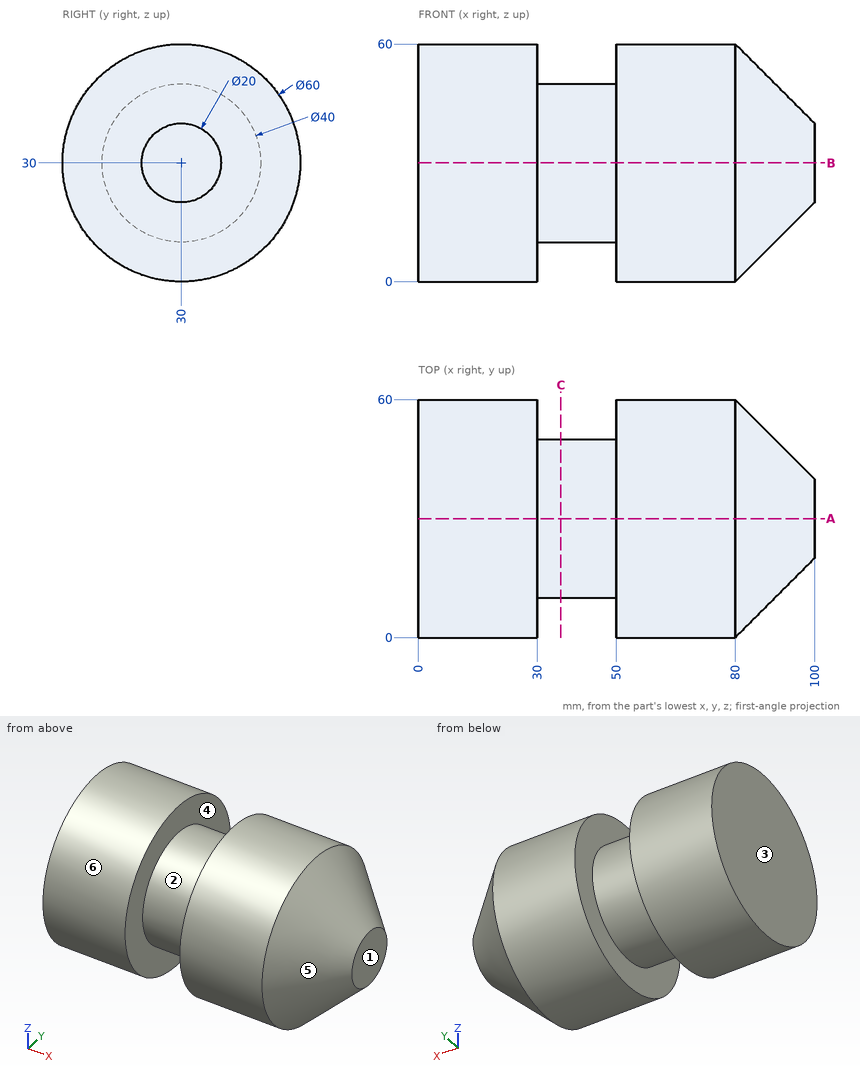
The figure shows three views and two pictorial views of one solid part (mm, origin at its lowest corner). Answer the questions. A direction names the side the tool comes from. Coordinates: 2 decimals unless noted, no trailing zeros. Write each loop counter-clockwise with the first axis right and the second up, starting at its lowest first coordinate (ties: lowest second). Pieces come first, ordered by that corner, then holes. Notation, with made-up numbers: (83.25, 14.25) -> (138.25, 14.25) arc R34 cw to (138.25, 45.25) -> close; hole circle Ø4 at (-26, 44). An arc over 180 degrees is marked (long way). Answer as a JSON object with one key per item and string values.
Q1. Determine the mould class of the marked faces 3, 4, 5 and 6 for opening direction X: pulls with the +X half, pulls with the -X half, needs draft (parallel to the pull), parting line crosses it, or undercut.
The answers:
{"face 3": "pulls with the -X half", "face 4": "undercut", "face 5": "pulls with the +X half", "face 6": "needs draft"}
Q2. The part is cut by section A-A on y = 30. Give the vertices of the cut face in (x, z), then the cut area to 3 significant figures.
The answers:
{"outline": "(0, 0) -> (30, 0) -> (30, 10) -> (50, 10) -> (50, 0) -> (80, 0) -> (100, 20) -> (100, 40) -> (80, 60) -> (50, 60) -> (50, 50) -> (30, 50) -> (30, 60) -> (0, 60) -> close", "area": "5,200 mm2"}
Q3. Flat-ended cylindrical pins translate along their axes: pin 1 Ø1.5 at (x, z) = (37, 33.5) entering from -Y; pin 2 Ø4 at (x, y) = (69, 20) entering from -Z; pin 3 Ø2 at (y, z) = (52, 27.5) entering from +X. Find the tip coordinate at first contact, or state that the pin passes through.
The answers:
{"pin 1": "stops at y = 10.19", "pin 2": "stops at z = 1.09", "pin 3": "stops at x = 88.86"}
Q4. The part is cut by section C-C on x = 36. Give the vertices of the cut face in (y, z).
The answers:
{"outline": "circle Ø40 at (30, 30)"}
Q5. A tool of negligible diameter and unlimited length cuts with its end or side. For the marked faces 1 and 2, from which of +Z, -Z, +X, -X, +Y, -Y can it reach the whole face along a straight path? Write none if from no direction.
The answers:
{"face 1": "+Z, -Z, +X, +Y, -Y", "face 2": "none"}
Q6. Consider line 1 (X direction, y = 4, z = 32); line 2 (X direction, y = 12.5, z = 52.5); line 3 (Y direction, x = 45, z = 39). Determine where each line is inside the solid, lowest interval first. Write a range as [from, to].
The answers:
{"line 1": "x = [0, 30], [50, 83.92]", "line 2": "x = [0, 30], [50, 81.5]", "line 3": "y = [12.14, 47.86]"}
